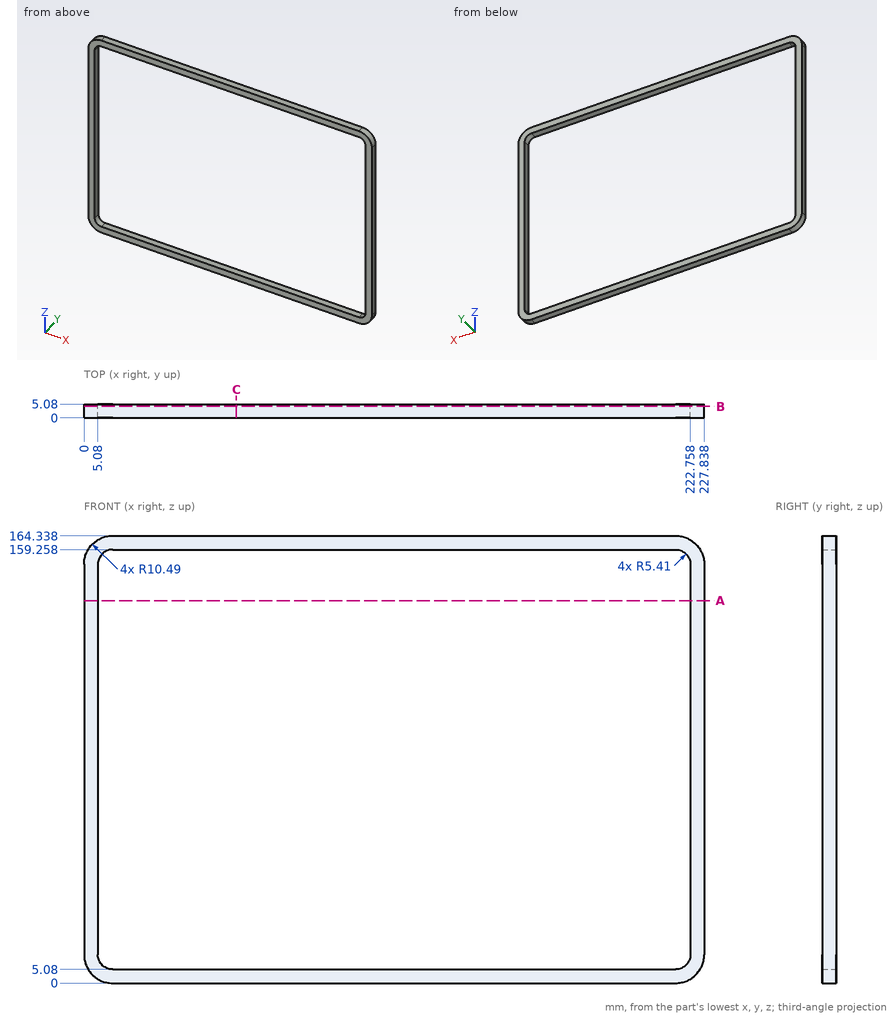
Study the drawing (mm; zero at the part's minimum x, y, z) and answer. Round coordinates to 2 decimals unless told otherwise and drop trailing zeros. Order: outer loops, then holes, each group sorted by start corner. A loop starts at its lowest first (then second) coordinate and runs counter-clockwise, first axis right, second up. Notation, with made-up numbers: (-5, 66) -> (35, 66) arc R9 cw to (35, 71) -> close; hole circle Ø7 at (81, -8.5). An arc over 180 degrees is marked (long way). Write each question's results on one line, items separated by ' | '. Start each with the question number.
Q1. Find section A-A (z = 140.5). Determine the outline of the cut face in (x, y), then the cut area to 3 significant figures.
Q2. Find section B-B (y = 4.2). Determine the outline of the cut face in (x, z).
Q3. Find section C-C (x = 56). Determine the outline of the cut face in (y, z), then the cut area to 3 significant figures.
Q4. Straight lines are drawn through the part: probe 1 along X at (y, z) = (2.1, 59); probe 2 along Z at (x, y) = (96, 4.25). For each, find the intervals that lie inside material, in ascending order. Write a range as from..to.
Worked answers:
1) outline: (0, 0) -> (5.08, 0) -> (5.08, 5.08) -> (0, 5.08) -> close; (222.76, 0) -> (227.84, 0) -> (227.84, 5.08) -> (222.76, 5.08) -> close | area: 51.6 mm2
2) outline: (0, 10.49) arc R10.49 ccw to (10.49, 0) -> (217.35, 0) arc R10.49 ccw to (227.84, 10.49) -> (227.84, 153.85) arc R10.49 ccw to (217.35, 164.34) -> (10.49, 164.34) arc R10.49 ccw to (0, 153.85) -> close; hole (5.08, 10.49) arc R5.41 ccw to (10.49, 5.08) -> (217.35, 5.08) arc R5.41 ccw to (222.76, 10.49) -> (222.76, 153.85) arc R5.41 ccw to (217.35, 159.26) -> (10.49, 159.26) arc R5.41 ccw to (5.08, 153.85) -> close
3) outline: (0, 0) -> (5.08, 0) -> (5.08, 5.08) -> (0, 5.08) -> close; (0, 159.26) -> (5.08, 159.26) -> (5.08, 164.34) -> (0, 164.34) -> close | area: 51.6 mm2
4) probe 1: x = 0..5.08, 222.76..227.84 | probe 2: z = 0..5.08, 159.26..164.34
